Could you check a few things on this model? Use its own coordinates, in mm. A direction names the side the tool comes from. Coordinates: 2 decimals unless noted, no trailing zeros. Write each loop counter-clockwise with the first axis right and the second up, starting at its lowest first coordinate (ties: lowest second). Pieces come first, ordered by that corner, then holes.
```python
from build123d import *

# Parameters (mm, degrees)
BOSS_EXTRUDE1_DEPTH   = 10
FILLET1_R             = 3
M3_TAPPED_HOLE2_D     = 2.5
M3_TAPPED_HOLE2_DEPTH = 15
M3_TAPPED_HOLE2_TIP   = 0.751075774


with BuildPart() as part:
    # Sketch1 → Boss-Extrude1 (new body)
    with BuildSketch(Plane.XY):
        Polygon((10, 10), (10, 0), (215, 0), (215, 10), (225, 10), (225, 85), (215, 85), (215, 95), (10, 95), (10, 85), (0, 85), (0, 10), align=None)
        with BuildLine():
            Line((20, 8), (55, 8))
            ThreePointArc((55, 8), (58, 5), (55, 2))
            Line((55, 2), (20, 2))
            ThreePointArc((20, 2), (17, 5), (20, 8))
        make_face(mode=Mode.SUBTRACT)
        with BuildLine():
            Line((65, 8), (100, 8))
            ThreePointArc((100, 8), (103, 5), (100, 2))
            Line((100, 2), (65, 2))
            ThreePointArc((65, 2), (62, 5), (65, 8))
        make_face(mode=Mode.SUBTRACT)
        with BuildLine():
            Line((3.5, 20), (3.5, 40))
            ThreePointArc((3.5, 40), (7.5, 44), (11.5, 40))
            Line((11.5, 40), (11.5, 20))
            ThreePointArc((11.5, 20), (7.5, 16), (3.5, 20))
        make_face(mode=Mode.SUBTRACT)
        with BuildLine():
            ThreePointArc((160, 8), (163, 5), (160, 2))
            Line((160, 2), (125, 2))
            ThreePointArc((125, 2), (122, 5), (125, 8))
            Line((125, 8), (160, 8))
        make_face(mode=Mode.SUBTRACT)
        with BuildLine():
            ThreePointArc((205, 8), (208, 5), (205, 2))
            Line((205, 2), (170, 2))
            ThreePointArc((170, 2), (167, 5), (170, 8))
            Line((170, 8), (205, 8))
        make_face(mode=Mode.SUBTRACT)
        with BuildLine():
            Line((213.5, 20), (213.5, 40))
            ThreePointArc((213.5, 40), (217.5, 44), (221.5, 40))
            Line((221.5, 40), (221.5, 20))
            ThreePointArc((221.5, 20), (217.5, 16), (213.5, 20))
        make_face(mode=Mode.SUBTRACT)
        with BuildLine():
            Line((3.5, 55), (3.5, 75))
            ThreePointArc((3.5, 75), (7.5, 79), (11.5, 75))
            Line((11.5, 75), (11.5, 55))
            ThreePointArc((11.5, 55), (7.5, 51), (3.5, 55))
        make_face(mode=Mode.SUBTRACT)
        with BuildLine():
            Line((20, 93), (55, 93))
            ThreePointArc((55, 93), (58, 90), (55, 87))
            Line((55, 87), (20, 87))
            ThreePointArc((20, 87), (17, 90), (20, 93))
        make_face(mode=Mode.SUBTRACT)
        with BuildLine():
            Line((65, 93), (100, 93))
            ThreePointArc((100, 93), (103, 90), (100, 87))
            Line((100, 87), (65, 87))
            ThreePointArc((65, 87), (62, 90), (65, 93))
        make_face(mode=Mode.SUBTRACT)
        Polygon((15, 63), (15, 85), (45, 85), align=None, mode=Mode.SUBTRACT)
        Polygon((15, 56.799641587), (53.455034199, 85), (171.544965801, 85), (210, 56.799641587), (210, 38.200358413), (171.544965801, 10), (53.455034199, 10), (15, 38.200358413), align=None, mode=Mode.SUBTRACT)
        Polygon((210, 32), (210, 10), (180, 10), align=None, mode=Mode.SUBTRACT)
        Polygon((180, 85), (210, 85), (210, 63), align=None, mode=Mode.SUBTRACT)
        Polygon((45, 10), (15, 10), (15, 32), align=None, mode=Mode.SUBTRACT)
        with BuildLine():
            Line((213.5, 55), (213.5, 75))
            ThreePointArc((213.5, 75), (217.5, 79), (221.5, 75))
            Line((221.5, 75), (221.5, 55))
            ThreePointArc((221.5, 55), (217.5, 51), (213.5, 55))
        make_face(mode=Mode.SUBTRACT)
        with BuildLine():
            Line((125, 93), (160, 93))
            ThreePointArc((160, 93), (163, 90), (160, 87))
            Line((160, 87), (125, 87))
            ThreePointArc((125, 87), (122, 90), (125, 93))
        make_face(mode=Mode.SUBTRACT)
        with BuildLine():
            Line((170, 93), (205, 93))
            ThreePointArc((205, 93), (208, 90), (205, 87))
            Line((205, 87), (170, 87))
            ThreePointArc((170, 87), (167, 90), (170, 93))
        make_face(mode=Mode.SUBTRACT)
    extrude(amount=BOSS_EXTRUDE1_DEPTH)

    # Fillet1
    fillet1_edges = [part.edges().sort_by_distance(p)[0] for p in [
        (15, 32, 5),
        (15, 10, 5),
        (45, 10, 5),
        (180, 10, 5),
        (210, 10, 5),
        (210, 32, 5),
        (210, 63, 5),
        (210, 85, 5),
        (180, 85, 5),
        (15, 85, 5),
        (15, 63, 5),
        (45, 85, 5),
        (53.455034199, 85, 5),
        (15, 56.799641587, 5),
        (15, 38.200358413, 5),
        (53.455034199, 10, 5),
        (171.544965801, 10, 5),
        (210, 38.200358413, 5),
        (210, 56.799641587, 5),
        (171.544965801, 85, 5),
    ]]
    fillet(fillet1_edges, radius=FILLET1_R)

    # M3 Tapped Hole2
    with Locations(Plane(origin=(0, 85, 0), x_dir=(1, 0, 0), z_dir=(0, 1, 0))):
        with Locations((220, -5), (5, -5)):
            Hole(M3_TAPPED_HOLE2_D / 2, depth=M3_TAPPED_HOLE2_DEPTH)
            with Locations((0, 0, -(M3_TAPPED_HOLE2_DEPTH + M3_TAPPED_HOLE2_TIP / 2))):  # 118° drill point
                Cone(0, M3_TAPPED_HOLE2_D / 2, M3_TAPPED_HOLE2_TIP, mode=Mode.SUBTRACT)


solid = part.part
```
1. On a 3-axis mill with a long thin cutter (end or side, diameter ignored), from which of +Z, -Z, +X, -X, +Y, -Y can I reach the whole of each face in a straight line? I mean faces 3 (the face through (5, 10, 5)), 4 (the face through (186.297, 12.117, 5.07)). Say none if no direction works.
Verdict:
face 3: +Z, -Z, -X, -Y
face 4: +Z, -Z
2. I want a section at C-C on y = 23.5. Please give me the cut outline in (x, z).
Verdict:
outline: (0, 0) - (3.5, 0) - (3.5, 10) - (0, 10) - close; (11.5, 0) - (15, 0) - (15, 10) - (11.5, 10) - close; (26.59, 0) - (35.05, 0) - (35.05, 10) - (26.59, 10) - close; (189.95, 0) - (198.41, 0) - (198.41, 10) - (189.95, 10) - close; (210, 0) - (213.5, 0) - (213.5, 10) - (210, 10) - close; (221.5, 0) - (225, 0) - (225, 10) - (221.5, 10) - close
3. For pin 1 (3 mm diameter, centred on x = 7.5, z = 5, fed in from +Y); pin 2 (3 mm diameter, centred on y = 92, z = 5.5, fed in from +X), each with a flat end and sliding along its axis, tell me the tip position at first contact or that it passes through.
Verdict:
pin 1: stops at y = 85
pin 2: stops at x = 215
4. I want a section at D-D on y = 35. Please give me the cut outline in (x, z).
Verdict:
outline: (0, 0) - (3.5, 0) - (3.5, 10) - (0, 10) - close; (11.5, 0) - (19.36, 0) - (19.36, 10) - (11.5, 10) - close; (205.64, 0) - (213.5, 0) - (213.5, 10) - (205.64, 10) - close; (221.5, 0) - (225, 0) - (225, 10) - (221.5, 10) - close
5. If we mould it in two halves opening along X, with no side actions, what happens to faces 1 (the face through (6, 85, 4)), 2 (the face through (7.4, 44, 4.9))? For each: pulls with the +X half, pulls with the -X half, needs draft (parallel to the pull), parting line crosses it, or undercut.
Verdict:
face 1: needs draft
face 2: undercut
6. I want a section at A-A on x = 110.5. Please give me the cut outline in (y, z), plus the area to 3 significant figures.
Verdict:
outline: (0, 0) - (10, 0) - (10, 10) - (0, 10) - close; (85, 0) - (95, 0) - (95, 10) - (85, 10) - close
area: 200 mm2
7. I want a section at B-B on y = 47.5. Please give me the cut outline in (x, z).
Verdict:
outline: (0, 0) - (15, 0) - (15, 10) - (0, 10) - close; (210, 0) - (225, 0) - (225, 10) - (210, 10) - close
8. Please list where these lines run through material, in increasing order: line 1 along Y through (x, z) = (54.5, 7.75); line 2 along X through (y, z) = (82.25, 5); line 3 along X through (y, z) = (34, 5).
Verdict:
line 1: y = 0 to 2, 8 to 10, 85 to 87, 93 to 95
line 2: x = 0 to 3.75, 6.25 to 15.01, 38.83 to 49.71, 175.29 to 186.17, 209.99 to 218.75, 221.25 to 225
line 3: x = 0 to 3.5, 11.5 to 20.73, 204.27 to 213.5, 221.5 to 225
